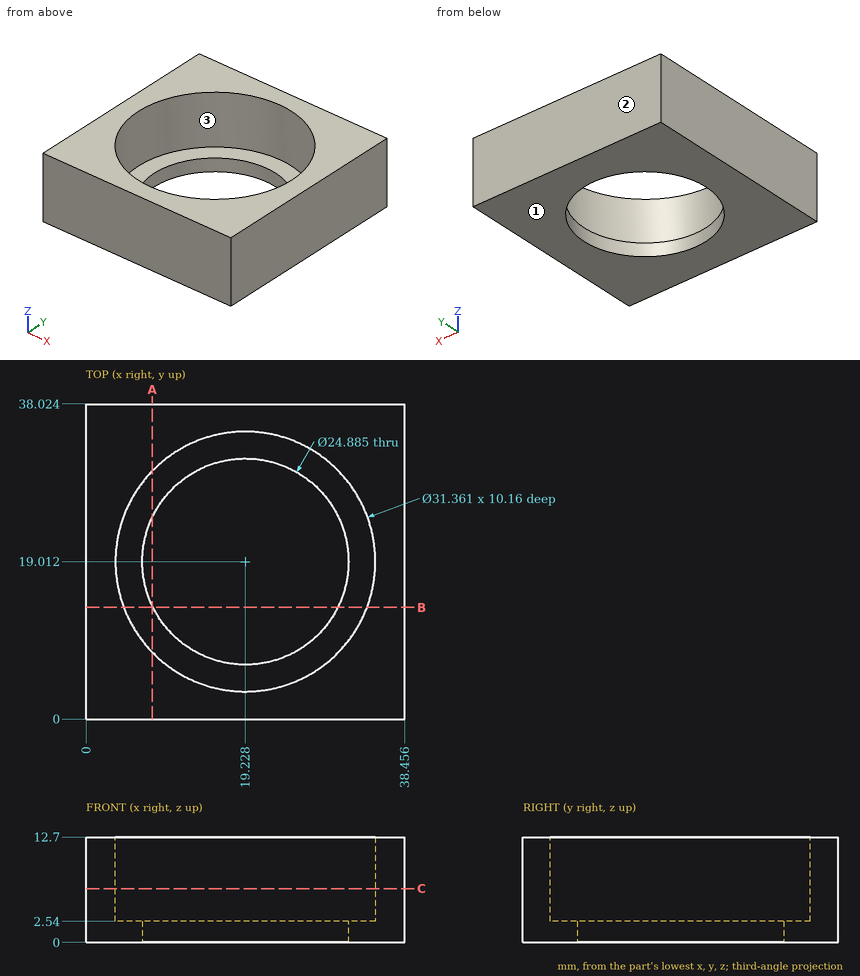
Job drawing, mm, ordinate dimensions from the low corner. One solid piece. Round coordinates to 2 decimals unless told otherwise and drop trailing zeros. Order: outer loops, then holes, each group sorted by start corner. A loop starts at its lowest first (then second) coordinate and runs counter-clockwise, first axis right, second up. Notation, with made-up numbers: (74, -8.75) -> (98, -8.75) arc R35 ccw to (98, 24.25) -> close; hole circle Ø7 at (1, 22.5). An arc over 180 degrees is marked (long way). Write item = value, one per line.
(1) Drill centre lines: L1, parallel to Y at x = 19, z = 4.5; L2, parallel to X at y = 24.5, z = 8.75 (1 decimal); L3, parallel to X at y = 23.5, z = 7.25 (1 decimal). Where is each one in solid material? Low to high.
Answers follow:
L1 = 0 to 3.33, 34.69 to 38.02
L2 = 0 to 4.5, 33.9 to 38.5
L3 = 0 to 4.2, 34.3 to 38.5
(2) Cut at B-B (y = 13.5). Write the cut outline in (x, z).
Answers follow:
outline = (0, 0) -> (8.07, 0) -> (8.07, 2.54) -> (4.55, 2.54) -> (4.55, 12.7) -> (0, 12.7) -> close; (30.38, 0) -> (38.46, 0) -> (38.46, 12.7) -> (33.91, 12.7) -> (33.91, 2.54) -> (30.38, 2.54) -> close
(3) Pull direction Y, two halves, no side cores. Call the marked faces 1, 2 and 3: +Y half, -Y half, draft (parallel to the pull), parting line (faces both ways), or undercut.
Answers follow:
face_1 = draft
face_2 = +Y half
face_3 = undercut
(4) Cut at A-A (x = 8). Write the cut outline in (y, z), plus the area to 3 significant figures.
Answers follow:
outline = (0, 0) -> (13.65, 0) -> (13.65, 2.54) -> (8.07, 2.54) -> (8.07, 12.7) -> (0, 12.7) -> close; (24.37, 0) -> (38.02, 0) -> (38.02, 12.7) -> (29.96, 12.7) -> (29.96, 2.54) -> (24.37, 2.54) -> close
area = 233 mm²
(5) Flat gauge pin, fed straight in: P1, Ø12, axis at x = 22.5, y = 24.5, coming from the -Z side. Where does the tip first touch, or does it go through?
Answers follow:
P1 = through
(6) Cut at C-C (z = 6.5). Write the cut outline in (x, y).
Answers follow:
outline = (0, 0) -> (38.46, 0) -> (38.46, 38.02) -> (0, 38.02) -> close; hole circle Ø31.36 at (19.23, 19.01)
